from build123d import *

# Parameters (mm, degrees)
SKETCH1_R           = 14.642304845
BOSS_EXTRUDE1_DEPTH = 2.5
BOSS_EXTRUDE2_DEPTH = 2.5
SKETCH3_R           = 4.25
BOSS_EXTRUDE3_DEPTH = 1.75
SKETCH4_R           = 2.1
CUT_EXTRUDE1_DEPTH  = 22.138984895
SKETCH5_R           = 2.6
CUT_EXTRUDE2_DEPTH  = 1.5
CUT_EXTRUDE3_REACH  = 23.78


with BuildPart() as part:
    # Sketch1 → Boss-Extrude1 (new body)
    with BuildSketch(Plane.XY):
        Circle(SKETCH1_R)
    extrude(amount=BOSS_EXTRUDE1_DEPTH)

    # Sketch2 → Boss-Extrude2 (add)
    with BuildSketch(Plane.XY.offset(2.5)):
        with BuildLine():
            Line((9.046191288, 11.513622991), (7.732334838, 8.140853638))
            ThreePointArc((7.732334838, 8.140853638), (2.22953316, 5.723381055), (-0.187939423, 11.226182734))
            Line((-0.187939423, 11.226182734), (1.125917027, 14.598952087))
            ThreePointArc((1.125917027, 14.598952087), (-9.158320976, 11.424633389), (-14.494185643, 2.077419967))
            Line((-14.494185643, 2.077419967), (-10.916353478, 2.625971582))
            ThreePointArc((-10.916353478, 2.625971582), (-6.071359969, -0.930858173), (-9.628189724, -5.775851681))
            Line((-9.628189724, -5.775851681), (-13.206021889, -6.324403296))
            ThreePointArc((-13.206021889, -6.324403296), (-5.314862256, -13.643655316), (5.447994356, -13.591042958))
            Line((5.447994356, -13.591042958), (3.18401864, -10.766825219))
            ThreePointArc((3.18401864, -10.766825219), (3.84182681, -4.792522882), (9.816129146, -5.450331052))
            Line((9.816129146, -5.450331052), (12.080104862, -8.274548791))
            ThreePointArc((12.080104862, -8.274548791), (14.473183232, 2.219021927), (9.046191288, 11.513622991))
        make_face()
    extrude(amount=BOSS_EXTRUDE2_DEPTH)

    # Sketch3 → Boss-Extrude3 (add)
    with BuildSketch(Plane.XY.offset(5)):
        with Locations(Location((0, 0, 0), (0, 0, 180))):
            Circle(SKETCH3_R)
    extrude(amount=BOSS_EXTRUDE3_DEPTH)

    # Sketch4 → Cut-Extrude1 (cut, through all)
    with BuildSketch(Plane.XY.offset(2.5)):
        with Locations((3.772197708, 9.683518186)):
            Circle(SKETCH4_R)
        with Locations((-10.272271601, -1.57494005)):
            Circle(SKETCH4_R)
        with Locations((6.500073893, -8.108578136)):
            Circle(SKETCH4_R)
    extrude(amount=-CUT_EXTRUDE1_DEPTH, mode=Mode.SUBTRACT)

    # Sketch5 → Cut-Extrude2 (cut)
    with BuildSketch(Plane.XY.offset(6.75)):
        Circle(SKETCH5_R)
    extrude(amount=-CUT_EXTRUDE2_DEPTH, mode=Mode.SUBTRACT)

    # Sketch6 → Cut-Extrude3 (cut, up to next)
    with BuildSketch(Plane.XY.offset(6.75), mode=Mode.PRIVATE) as cut_extrude3_sk1:
        with BuildLine():
            Line((-1.65, 2.00935313), (-1.65, -2.00935313))
            ThreePointArc((-1.65, -2.00935313), (0, -2.6), (1.65, -2.00935313))
            Line((1.65, -2.00935313), (1.65, 2.00935313))
            ThreePointArc((1.65, 2.00935313), (0, 2.6), (-1.65, 2.00935313))
        make_face()
    cut_extrude3_tool1 = extrude(cut_extrude3_sk1.sketch, amount=-CUT_EXTRUDE3_REACH, mode=Mode.PRIVATE) & part.part
    add(cut_extrude3_tool1.solids().sort_by_distance((0, 0, 6.75))[0], mode=Mode.SUBTRACT)


solid = part.part
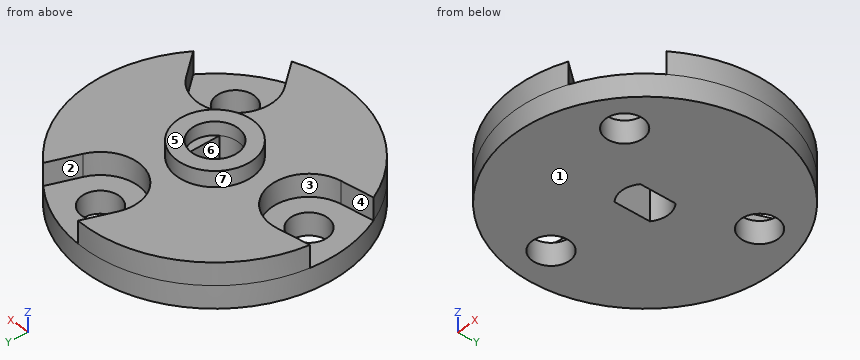
For this review, take the finished solid that the model builds, in its own axes (mm). Face numbers are marked on the shaded views. A direction names the side the tool comes from. Round coordinates to 2 decimals unless told otherwise and drop trailing zeros. Write each loop counter-clockwise with the first axis right and the second up, starting at its lowest first coordinate (ties: lowest second). Pieces come first, ordered by that corner, then holes. Notation, with made-up numbers: (-33, 87.25) - (13, 87.25) arc R19 cw to (13, 117.25) - close; hole circle Ø8 at (-12.5, 11.25). An arc over 180 degrees is marked (long way). Write item = value, one per line. Start each with the question number.
1. Consider section B-B on y = 0. State the section outline as (x, z) points, plus the area to 3 significant figures.
2. For the marked faces 5, 6 and 7, list the 3-axis set-ups (+Z, -Z, +X, -X, +Y, -Y) from which the entire face can be reached by the end or side of a thin tool; tool diameter is ignored.
3. Wall thickness on L1, parallel to Z at x = 8, y = 1.75; L2, parallel to Z at x = 1.75, y = 10.5; L3, parallel to Y at x = 3, z = 1: over which ranges is each line inside the solid? List them lowest first.
4. Consider section A-A on z = 3.75. State the section outline as (x, y) points, plus the area to 3 significant figures.
5. For pin 1 Ø1 at (x, y) = (2, -0.5) entering from +Z; pin 2 Ø6.5 at (x, y) = (-10.27, -1.57) entering from +Z; pin 3 Ø1 at (x, z) = (4.5, 3.5) entering from +Y, all flat-tipped, find the tip position at first contact; note any pin that passes through.
6. Consider section C-C on x = 11. State the section outline as (y, z) points.
7. Consider section D-D on z = 1.5. State the section outline as (x, y) points.
8. Draft analysis for pull direction X (two halves, no side actions). For the marked faces 1, 2, 3 and 4, state which applies: released by +X, released by -X, zero draft, split by the parting line, or undercut.
Evaluation:
q1.outline = (-14.64, 0) - (-11.66, 0) - (-11.66, 2.5) - (-14.64, 2.5) - close; (-8.88, 0) - (-1.65, 0) - (-1.65, 5.25) - (-2.6, 5.25) - (-2.6, 6.75) - (-4.25, 6.75) - (-4.25, 5) - (-6.32, 5) - (-6.32, 2.5) - (-8.88, 2.5) - close; (1.65, 0) - (14.64, 0) - (14.64, 5) - (4.25, 5) - (4.25, 6.75) - (2.6, 6.75) - (2.6, 5.25) - (1.65, 5.25) - close
q1.area = 108 mm2
q2.face_5 = +Z, +X, -X, +Y, -Y
q2.face_6 = +Z, -Z
q2.face_7 = +Z
q3.L1 = 0 to 5
q3.L2 = 0 to 2.5
q3.L3 = -14.33 to 7.73, 11.64 to 14.33
q4.outline = (-14.49, 2.08) - (-10.92, 2.63) arc R4.25 cw to (-9.63, -5.78) - (-13.21, -6.32) arc R14.64 ccw to (5.45, -13.59) - (3.18, -10.77) arc R4.25 cw to (9.82, -5.45) - (12.08, -8.27) arc R14.64 ccw to (9.05, 11.51) - (7.73, 8.14) arc R4.25 cw to (-0.19, 11.23) - (1.13, 14.6) arc R14.64 ccw to start; hole (-1.65, -2.01) arc R2.6 ccw to (1.65, -2.01) - (1.65, 2.01) arc R2.6 ccw to (-1.65, 2.01) - close
q4.area = 469 mm2
q5.pin_1 = 5.25
q5.pin_2 = 2.5
q5.pin_3 = 5.61
q6.outline = (-9.66, 0) - (9.66, 0) - (9.66, 5) - (-6.93, 5) - (-6.93, 2.5) - (-9.66, 2.5) - close
q7.outline = circle Ø29.28 at (0, 0); hole circle Ø4.2 at (-10.27, -1.57); hole (-1.65, -2.01) arc R2.6 ccw to (1.65, -2.01) - (1.65, 2.01) arc R2.6 ccw to (-1.65, 2.01) - close; hole circle Ø4.2 at (3.77, 9.68); hole circle Ø4.2 at (6.5, -8.11)
q8.face_1 = zero draft
q8.face_2 = undercut
q8.face_3 = undercut
q8.face_4 = released by -X
